The listing builds one solid part. Answer for the finished solid, in the listing's coordinates (mm). A direction names the side the tool comes from. Round coordinates to 2 decimals unless told otherwise and drop trailing zeros. Order: outer loops, then holes, each group sorted by start corner. A loop starts at its lowest first (then second) coordinate and runs counter-clockwise, first axis right, second up. Notation, with made-up numbers: (-28, 9.25) -> (4, 9.25) arc R20 ccw to (4, 18.25) -> close; hole circle Ø4 at (23.5, 19.5). An arc over 180 degrees is marked (long way). Return JSON: item names as keys, results as strings. Group by question number.
(1) The part is cut by section D-D (z = 4). Determine the outline of the cut face in (x, y), plus the area to 3 significant figures.
(2) Each of these flat-tipped pins is pushed along its axis until it touches: pin 1 (4 mm diameter, centred on x = 2.5, z = -7.5, fed in from -Y); pin 2 (2 mm diameter, centred on y = 3, z = 7, fed in from +X). Where does it stop, or does it pass through?
(3) The part is cut by section B-B (y = 4.2). Count the separate pieces of the cut face and the enclosed holes in it, plus the area to 3 significant figures.
(4) Which of the six approach directions +Z, -Z, +X, -X, +Y, -Y give full straight-line access (tool end or side, diameter ignored) to faces 5 (the face through (-7.5, 2, 7)), 6 (the face through (9.5, 2, -3)), 7 (the face through (7.5, 2, 6))?
(5) Consider line 1 (X direction, y = 3.15, z = -6.8); line 2 (X direction, y = 3.1, z = -7.25); line 3 (X direction, y = 1.95, z = 8.25). Determine where each line is inside the solid, lowest interval first. Write a range as [from, to].
(6) The part is cut by section C-C (x = -6.8). Determine the outline of the cut face in (y, z).
(7) Determine the mould class of faces 1 (the face through (-7.183, 2.465, -5.876)), 2 (the face through (7.801, 2.535, 3.785)), 3 (the face through (0, 2, -9.5)), 4 (the face through (0, 0, 0)) for opening direction Z: +Z half, -Z half, draft (parallel to the pull), parting line (faces both ways), or undercut.
(8) The part is cut by section A-A (z = -6.8). Determine the outline of the cut face in (x, y), plus the area to 3 significant figures.
from build123d import *

# Parameters (mm, degrees)
ESQUISSE2_R        = 1
BOSS_EXTRU_1_DEPTH = 5
CONG_1_R           = 1


with BuildPart() as part:
    # Esquisse2 → Boss.-Extru.1 (new body)
    with BuildSketch(Plane(origin=(0, 0, 0), x_dir=(1, 0, 0), z_dir=(0, 1, 0))):
        Polygon((-9.5, -3.5), (-9.5, 9.5), (9.5, 9.5), (9.5, -3.5), (7.5, -3.5), (7.5, -9.5), (-7.5, -9.5), (-7.5, -3.5), align=None)
        with Locations(Location((-6.8, 6.8, 0), (0, 0, 270))):
            Circle(ESQUISSE2_R, mode=Mode.SUBTRACT)
        with Locations(Location((6.8, 6.8, 0), (0, 0, 90))):
            Circle(ESQUISSE2_R, mode=Mode.SUBTRACT)
    extrude(amount=BOSS_EXTRU_1_DEPTH)

    # Congé1
    cong_1_edges = [part.edges().sort_by_distance(p)[0] for p in [
        (9.5, 2.5, -9.5),
        (9.5, 2.5, 3.5),
        (7.5, 2.5, 3.5),
        (7.5, 2.5, 9.5),
        (-7.5, 2.5, 9.5),
        (-7.5, 2.5, 3.5),
        (-9.5, 2.5, 3.5),
        (-9.5, 2.5, -9.5),
    ]]
    fillet(cong_1_edges, radius=CONG_1_R - 0.0001)  # a hair under: the kernel refuses the full size


solid = part.part
Answer below:
{
 "1": {"outline": "(-7.63, 0) -> (7.63, 0) -> (7.63, 5) -> (-7.63, 5) -> close", "area": "76.3 mm²"},
 "2": {"pin 1": "stops at y = 0", "pin 2": "stops at x = 7.5"},
 "3": {"separate pieces": "1", "enclosed holes": "2", "area": "330 mm²"},
 "4": {"face 5": "+Z, -X, +Y, -Y", "face 6": "+Z, -Z, +X, +Y, -Y", "face 7": "+Z, +X, +Y, -Y"},
 "5": {"line 1": "x = [-9.5, -7.8], [-5.8, 5.8], [7.8, 9.5]", "line 2": "x = [-9.5, -7.69], [-5.91, 5.91], [7.69, 9.5]", "line 3": "x = [-7.5, 7.5]"},
 "6": {"outline": "(0, -9.5) -> (5, -9.5) -> (5, -7.8) -> (0, -7.8) -> close; (0, -5.8) -> (5, -5.8) -> (5, 9.45) -> (0, 9.45) -> close"},
 "7": {"face 1": "undercut", "face 2": "+Z half", "face 3": "-Z half", "face 4": "draft"},
 "8": {"outline": "(-9.5, 0) -> (-7.8, 0) -> (-7.8, 5) -> (-9.5, 5) -> close; (-5.8, 0) -> (5.8, 0) -> (5.8, 5) -> (-5.8, 5) -> close; (7.8, 0) -> (9.5, 0) -> (9.5, 5) -> (7.8, 5) -> close", "area": "75.0 mm²"}
}
